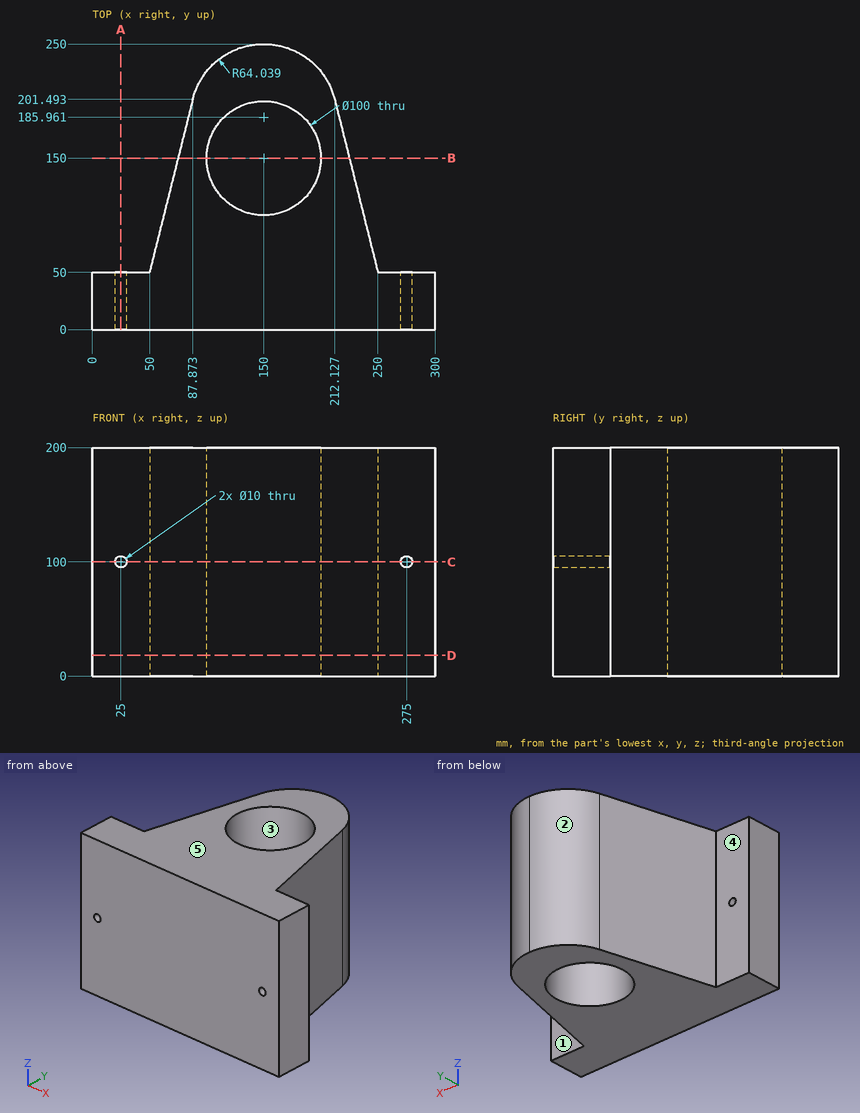
Design review of the part shown in the three views and the two pictorial views. Dimensions are in mm from the part's minimum x, y and z. A direction names the side the tool comes from. Coordinates: 2 decimals unless noted, no trailing zeros. Order: outer loops, then holes, each group sorted by start corner. A loop starts at its lowest first (then second) coordinate and runs counter-clockwise, first axis right, second up. Notation, with made-up numbers: (-7, 53.25) - (17, 53.25) arc R33 cw to (17, 87.25) - close; hole circle Ø4 at (0, 24). An arc over 180 degrees is marked (long way). One line per question, with ' | ' between items.
Q1. To check wall thickness, follow line 1 along X through (y, z) = (12, 100); line 2 along Z through (x, y) = (275, 16); line 3 along Y through (x, z) = (40, 44). State the ranges of each line that lie inside material, in increasing order.
Answer key:
line 1: x = 0 to 20, 30 to 270, 280 to 300 | line 2: z = 0 to 95, 105 to 200 | line 3: y = 0 to 50
Q2. Consider section D-D, the plane z = 18. Give the boundary of the cut face in (x, y), then the cut area to 3 significant figures.
Answer key:
outline: (0, 0) - (300, 0) - (300, 50) - (250, 50) - (212.13, 201.49) arc R64.04 ccw to (87.87, 201.49) - (50, 50) - (0, 50) - close; hole circle Ø100 at (150, 150) | area: 36,200 mm2
Q3. The part is to be moulded in two halves that separate along Y. For the marked faces 3, 4 and 5, say which applies: +Y half, -Y half, draft (parallel to the pull), parting line (faces both ways), or undercut.
Answer key:
face 3: undercut | face 4: +Y half | face 5: draft
Q4. Consider section B-B, the plane y = 150. Give the boundary of the cut face in (x, z).
Answer key:
outline: (75, 0) - (100, 0) - (100, 200) - (75, 200) - close; (200, 0) - (225, 0) - (225, 200) - (200, 200) - close
Q5. Consider section C-C, the plane z = 100. Give the boundary of the cut face in (x, y), then the cut area to 3 significant figures.
Answer key:
outline: (0, 0) - (20, 0) - (20, 50) - (0, 50) - close; (30, 0) - (270, 0) - (270, 50) - (250, 50) - (212.13, 201.49) arc R64.04 ccw to (87.87, 201.49) - (50, 50) - (30, 50) - close; (280, 0) - (300, 0) - (300, 50) - (280, 50) - close; hole circle Ø100 at (150, 150) | area: 35,200 mm2
Q6. Clearance check with flat-ended pins moving along their axes: pin 1 Ø6 at (x, z) = (275, 100) entering from +Y; pin 2 Ø2 at (y, z) = (163.5, 79) entering from -X (3 decimals); pin 3 Ø1 at (x, z) = (198, 92.5) entering from -Y; pin 4 Ø12 at (y, z) = (177.5, 134.5) entering from +X (3 decimals). State where each tip first meets the part, or that it passes through.
Answer key:
pin 1: passes through | pin 2: stops at x = 78.125 | pin 3: stops at y = 0 | pin 4: stops at x = 219.625
Q7. Consider section A-A, the plane x = 25. Give the boundary of the cut face in (y, z).
Answer key:
outline: (0, 0) - (50, 0) - (50, 95) - (0, 95) - close; (0, 105) - (50, 105) - (50, 200) - (0, 200) - close
Q8. For the marked faces 1 and 2, list the 3-axis set-ups (+Z, -Z, +X, -X, +Y, -Y) from which the entire face can be reached by the end or side of a thin tool; tool diameter is ignored.
Answer key:
face 1: +Z, -Z, +X, +Y | face 2: +Z, -Z, -X, +Y
